```python
from build123d import *

# Parameters (mm, degrees)
SKETCH1_W                       = 225.425
SKETCH1_H                       = 225.425
SKETCH1_W_2                     = 202.565
SKETCH1_H_2                     = 202.565
BOSS_EXTRUDE1_DEPTH             = 25.4
TAP_DRILL_FOR_1_4_20_TAP1_D     = 5.1054
TAP_DRILL_FOR_1_4_20_TAP1_DEPTH = 12.7
TAP_DRILL_FOR_1_4_20_TAP1_TIP   = 1.533816902


with BuildPart() as part:
    # Sketch1 → Boss-Extrude1 (new body)
    with BuildSketch(Plane(origin=(0, 0, 0), x_dir=(1, 0, 0), z_dir=(0, 1, 0))):
        with Locations((112.7125, -112.7125)):
            Rectangle(SKETCH1_W, SKETCH1_H)
        with Locations((112.7125, -112.7125)):
            Rectangle(SKETCH1_W_2, SKETCH1_H_2, mode=Mode.SUBTRACT)
    extrude(amount=BOSS_EXTRUDE1_DEPTH)

    # Tap Drill for 1/4-20 Tap1
    with Locations(Plane(origin=(0, 25.4, 0), x_dir=(1, 0, 0), z_dir=(0, 1, 0))):
        with Locations((25.4, -5.715), (50.8, -5.715), (76.2, -5.715), (101.6, -5.715), (127, -5.715), (152.4, -5.715), (177.8, -5.715), (203.2, -5.715), (5.715, -25.4), (5.715, -50.8), (5.715, -76.2), (5.715, -101.6), (5.715, -127), (5.715, -152.4), (5.715, -177.8), (5.715, -203.2), (219.71, -22.225), (219.71, -47.625), (219.71, -73.025), (219.71, -98.425), (219.71, -123.825), (219.71, -149.225), (219.71, -174.625), (219.71, -200.025), (22.225, -219.71), (47.625, -219.71), (73.025, -219.71), (98.425, -219.71), (123.825, -219.71), (149.225, -219.71), (174.625, -219.71), (200.025, -219.71)):
            Hole(TAP_DRILL_FOR_1_4_20_TAP1_D / 2, depth=TAP_DRILL_FOR_1_4_20_TAP1_DEPTH)
            with Locations((0, 0, -(TAP_DRILL_FOR_1_4_20_TAP1_DEPTH + TAP_DRILL_FOR_1_4_20_TAP1_TIP / 2))):  # 118° drill point
                Cone(0, TAP_DRILL_FOR_1_4_20_TAP1_D / 2, TAP_DRILL_FOR_1_4_20_TAP1_TIP, mode=Mode.SUBTRACT)


solid = part.part
```
CAD build for the part. Positions are in the model's coordinates, mm. A direction names the side the tool comes from. Coordinates: 2 decimals unless noted, no trailing zeros. Order: outer loops, then holes, each group sorted by start corner. A loop starts at its lowest first (then second) coordinate and runs counter-clockwise, first axis right, second up. Notation, with made-up numbers: (39.5, 74.25) - (70.5, 74.25) arc R31 ccw to (70.5, 104.25) - close; hole circle Ø11 at (83, -21.5). An arc over 180 degrees is marked (long way). Answer in a Markdown table with one row per item.
1. Slice it at B-B, the plane x = 34. List the corners of the cut face in (y, z) (3 decimals), then the cut area to 3 significant figures.
Answer:
| item | result |
|---|---|
| outline | (0, 0) - (25.4, 0) - (25.4, 11.43) - (0, 11.43) - close; (0, 213.995) - (25.4, 213.995) - (25.4, 225.425) - (0, 225.425) - close |
| area | 581 mm² |
2. Drill centre lines: L1, parallel to X at y = 17, z = 203.2 (3 decimals); L2, parallel to Z at x = 160, y = 22.5 (3 decimals). Where is each one in solid material? Low to high. Write a range as from..to.
Answer:
| item | result |
|---|---|
| L1 | 0..3.162, 8.268..11.43, 213.995..225.425 |
| L2 | 0..11.43, 213.995..225.425 |
3. Pull direction Z, two halves, no side cores. Call faces 1 (the face through (220.13, 11.43, 72.89)), 2 (the face through (4.537, 18.961, 53.065)): +Z half, -Z half, draft (parallel to the pull), parting line (faces both ways), or undercut.
Answer:
| item | result |
|---|---|
| face 1 | undercut |
| face 2 | undercut |
4. Slice it at C-C, the plane y = 4. List the corners of the cut face in (x, z) (3 decimals), then the cut area to 3 significant figures.
Answer:
| item | result |
|---|---|
| outline | (0, 0) - (225.425, 0) - (225.425, 225.425) - (0, 225.425) - close; hole (11.43, 11.43) - (213.995, 11.43) - (213.995, 213.995) - (11.43, 213.995) - close |
| area | 9,780 mm² |
5. Slice it at D-D, the plane y = 19. Give the number of separate pieces and of enclosed holes in the cut face, then the cut area to 3 significant figures.
Answer:
| item | result |
|---|---|
| separate pieces | 1 |
| enclosed holes | 33 |
| area | 9,130 mm² |
6. Flat gauge pin, fed straight in: P1, Ø4, axis at x = 76.2, z = 5.715, coming from the +Y side. Where does the tip first touch, or does it go through?
Answer:
| item | result |
|---|---|
| P1 | y = 12.37 |
7. Slice it at A-A, the plane z = 58. List the corners of the cut face in (x, y) (3 decimals).
Answer:
| item | result |
|---|---|
| outline | (0, 0) - (11.43, 0) - (11.43, 25.4) - (0, 25.4) - close; (213.995, 0) - (225.425, 0) - (225.425, 25.4) - (213.995, 25.4) - close |
8. 3-axis set-ups, long thin cutter, end or side, ignore diameter. For faces 3 (the face through (213.995, 13, 114)), 4 (the face through (217.275, 18.961, 199.258)): which of +Z, -Z, +X, -X, +Y, -Y reach the whole face in a straight line?
Answer:
| item | result |
|---|---|
| face 3 | +Y, -Y |
| face 4 | +Y |
